Study the drawing (mm; zero at the part's minimum x, y, z) and answer. A direction names the side the tool comes from. Coordinates: 2 decimals unless noted, no trailing zeros. Order: outer loops, then holes, each group sorted by start corner. A loop starts at its lowest first (then second) coordinate and runs counter-clockwise, first axis right, second up.
1. Find the intervals of material crossed by probe 1 along X at (y, z) = (27, 36); probe 2 along Z at (x, y) = (103.5, 46.5); probe 3 along Y at (x, z) = (25, 9), in increasing order.
2. The part is cut by section B-B, the plane x = 96. Give the vertices of the cut face in (y, z), then the cut area to 3 significant figures.
3. A tool of negligible diameter and unlimited length cuts with its end or side. For the marked faces 5, 6 and 7, from which of +Z, -Z, +X, -X, +Y, -Y can it reach the whole face along a straight path? Write none if from no direction.
4. Determine the mould class of the marked faces 1, 2, 3 and 4 for opening direction X: +X half, -X half, draft (parallel to the pull), parting line (faces both ways), or undercut.
5. The part is cut by section D-D, the plane z = 41.5. Give the vertices of the cut face in (x, y), then the cut area to 3 significant figures.
6. Flat-ended cylindrical pins translate along their axes: pin 1 Ø7 at (x, y) = (96, 38) entering from +Z; pin 2 Ø2.5 at (x, y) = (108, 62.5) entering from -Z; pin 3 Ø8 at (y, z) = (41, 42) entering from -X. Find the tip coordinate at first contact, or state that the pin passes through.
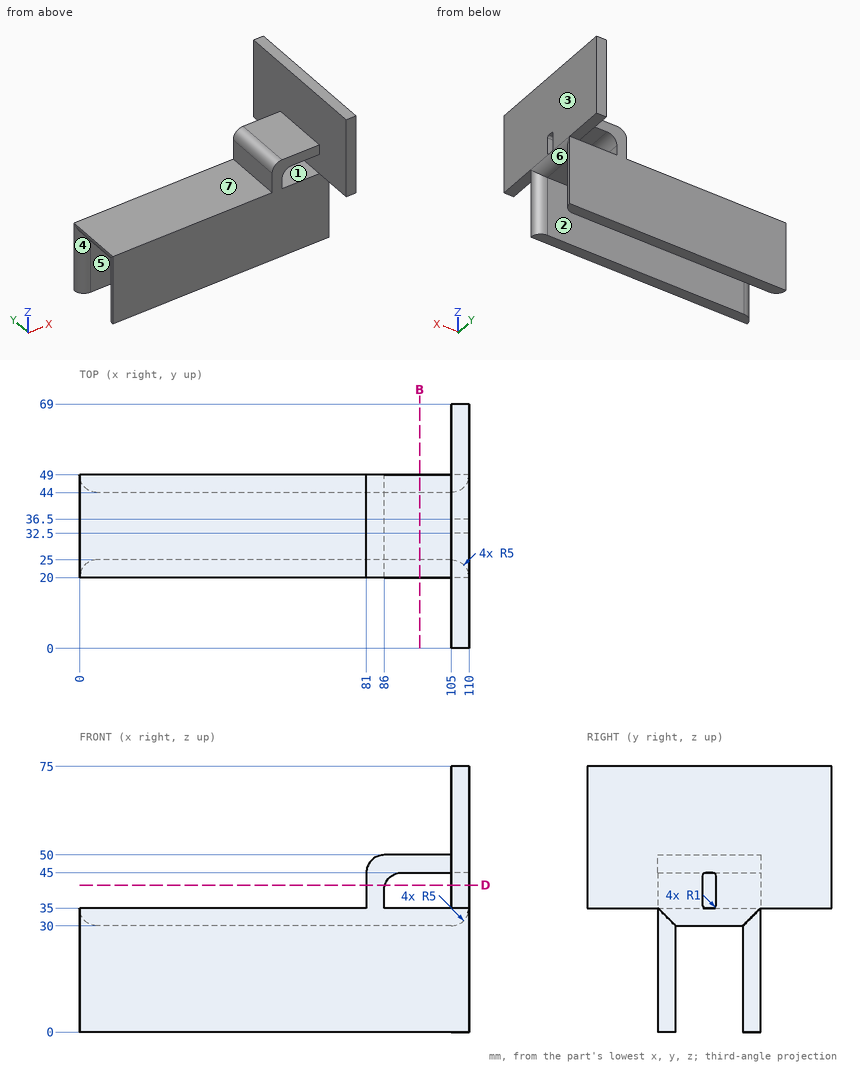
Geometry says:
1. probe 1: x = 81 to 86, 105 to 110
1. probe 2: z = 0 to 35, 45 to 50
1. probe 3: y = 20 to 25, 44 to 49
2. outline: (20, 0) - (25, 0) - (25, 30) - (44, 30) - (44, 0) - (49, 0) - (49, 35) - (20, 35) - close; (20, 45) - (49, 45) - (49, 50) - (20, 50) - close
2. area: 590 mm2
3. face 5: -Z, +X, -X
3. face 6: -Z, +X
3. face 7: +Z, -X, +Y, -Y
4. face 1: undercut
4. face 2: draft
4. face 3: +X half
4. face 4: -X half
5. outline: (81, 20) - (86.23, 20) - (86.23, 49) - (81, 49) - close; (105, 0) - (110, 0) - (110, 32.5) - (105, 32.5) - close; (105, 36.5) - (110, 36.5) - (110, 69) - (105, 69) - close
5. area: 477 mm2
6. pin 1: stops at z = 50
6. pin 2: stops at z = 35
6. pin 3: stops at x = 81
